For this review, take the finished solid that the model builds, in its own axes (mm). A direction names the side the tool comes from. Round coordinates to 2 decimals unless told otherwise and drop trailing zeros. Order: outer loops, then holes, each group sorted by start corner. A loop starts at its lowest first (then second) coordinate and runs counter-clockwise, first axis right, second up. Notation, with made-up numbers: (36, 85) -> (70, 85) arc R34 ccw to (70, 115) -> close; hole circle Ø4 at (-27.75, 73.5). An arc over 180 degrees is marked (long way). Use a Markdown table: item, result. Add a question column.
1) Consider section A-A (y = 7.5). State the section outline as (x, z) points (3 decimals).
2) Machinability: for faces 1 (the face through (-12, 3, -4)), 2 (the face through (-7, 2, -6.542)), 3 (the face through (10.318, 2.217, -6.705)), 4 (the face through (12, 3, -4)), 5 (the face through (10.27, 0.72, -4.52)), which of the approach directions +Z, -Z, +X, -X, +Y, -Y give a long, thin tool a straight path to every point of the face, cutting with its end or side? Answer none if there is none.
3) Clearance check with flat-ended pins moving along their axes: P1, Ø1.1, axis at x = 7, z = -4.5, coming from the -Y side; P2, Ø0.7, axis at x = 8, y = 1, coming from the +Z side; P3, Ø4.5, axis at x = 10, z = -5.5, coming from the +Y side; P4, Ø1, axis at x = -6.5, z = -1, coming from the -Y side. State where each tip first meets the part, or that it passes through.
4) Wall thickness on line 1 along X through (y, z) = (2.25, 1.25) (3 decimals); line 2 along Y through (x, z) = (3.25, 3.25); line 3 along Z through (x, y) = (8.75, 1): over which ranges is each line inside the solid? List them lowest first. Write a range as [from, to].
5) Consider section B-B (z = -4.55). Give the number of separate pieces and of enclosed holes in the cut face, plus the area to 3 significant figures.
6) Draft analysis for pull direction Z (two halves, no side actions). For faces 6 (the face through (-7.93, 3.45, -1.26)), 7 (the face through (8, 1, -5.82)), 8 (the face through (-13.3, 1.5, -4.6)), state which applies: pulls with the +Z half, pulls with the -Z half, needs draft (parallel to the pull), parting line crosses it, or undercut.
7) Consider section C-C (z = 4). State the section outline as (x, y) points (3 decimals).
8) Consider section D-D (x = 2.25). State the section outline as (y, z) points, plus the area to 4 significant figures.
```python
from build123d import *

# Parameters (mm, degrees)
SKETCH1_W          = 15
SKETCH1_H          = 17.3
EXTRUDE1_DEPTH     = 11.5
SKETCH2_W          = 12.15
SKETCH2_H          = 10
EXTRUDE2_DEPTH     = 17.3
EXTRUDE3_DEPTH     = 3
CUT_EXTRUDE3_DEPTH = 1.5875
CUT_EXTRUDE1_DEPTH = 18.998958303
FILLET3_R          = 1.5
FILLET1_R          = 1.5


with BuildPart() as part:
    # Sketch1 → Extrude1 (new body)
    with BuildSketch(Plane(origin=(0, 0, 0), x_dir=(1, 0, 0), z_dir=(0, 1, 0))):
        Rectangle(SKETCH1_W, SKETCH1_H)
    extrude(amount=EXTRUDE1_DEPTH)

    # Sketch2 → Extrude2 (cut)
    with BuildSketch(Plane.XY.offset(8.65)):
        with Locations((0, 5)):
            Rectangle(SKETCH2_W, SKETCH2_H)
    extrude(amount=-EXTRUDE2_DEPTH, mode=Mode.SUBTRACT)

    # Sketch3 → Extrude3 (add)
    with BuildSketch(Plane.XZ):
        with BuildLine():
            Line((7.5, -8.65), (10.169151464, -8.65))
            ThreePointArc((10.169151464, -8.65), (13.3, -4.55), (10.169151464, -0.45))
            Line((10.169151464, -0.45), (7.5, -0.45))
            Line((7.5, -0.45), (7.5, -8.65))
        make_face()
    extrude3 = extrude(amount=-EXTRUDE3_DEPTH)

    # Sketch8 → Cut-Extrude3 (cut)
    with BuildSketch(Plane(origin=(0, 3, 0), x_dir=(-1, 0, 0), z_dir=(0, 1, 0))):
        Polygon((-11.55, -5.993375673), (-9.05, -7.436751346), (-6.55, -5.993375673), (-6.55, -3.106624327), (-9.05, -1.663248654), (-11.55, -3.106624327), align=None)
    cut_extrude3 = extrude(amount=-CUT_EXTRUDE3_DEPTH, mode=Mode.SUBTRACT)

    # Sketch5 → Cut-Extrude1 (cut, through all)
    with BuildSketch(Plane.XZ.offset(-3)):
        with BuildLine():
            Line((9, -5.82), (7.5, -5.82))
            Line((7.5, -5.82), (7.5, -6.541858429))
            Line((7.5, -6.541858429), (6.075, -6.541858429))
            Line((6.075, -6.541858429), (6.075, -2.558141571))
            Line((6.075, -2.558141571), (7.5, -2.558141571))
            Line((7.5, -2.558141571), (7.5, -3.28))
            Line((7.5, -3.28), (9, -3.28))
            ThreePointArc((9, -3.28), (10.27, -4.55), (9, -5.82))
        make_face()
    cut_extrude1 = extrude(amount=CUT_EXTRUDE1_DEPTH, mode=Mode.SUBTRACT)

    # Mirror3: Extrude3, Cut-Extrude3, Cut-Extrude1 across plane
    add(extrude3.mirror(Plane(origin=(0, 0, 0), x_dir=(0, 0, 1), z_dir=(1, 0, 0))))
    add(cut_extrude3.mirror(Plane(origin=(0, 0, 0), x_dir=(0, 0, 1), z_dir=(1, 0, 0))), mode=Mode.SUBTRACT)
    add(cut_extrude1.mirror(Plane(origin=(0, 0, 0), x_dir=(0, 0, 1), z_dir=(1, 0, 0))), mode=Mode.SUBTRACT)

    # Fillet3
    fillet3_edges = [part.edges().sort_by_distance(p)[0] for p in [
        (-7.5, 11.5, 0),
        (7.5, 11.5, 0),
    ]]
    fillet(fillet3_edges, radius=FILLET3_R)

    # Fillet1
    # the kernel refuses this fillet: 1.5 mm, written as the material it adds along each edge
    with BuildSketch(Plane(origin=(7.5, 3, -0.45), x_dir=(0, 1, 0), z_dir=(0, 0, -1))) as fillet1_piece_1_section:
        with BuildLine():
            CenterArc((FILLET1_R, FILLET1_R), FILLET1_R, 180, 90)
            Line((0, FILLET1_R), (0, 0))
            Line((0, 0), (FILLET1_R, 0))
        make_face()
    fillet1_piece_1 = extrude(amount=5.858141571, mode=Mode.PRIVATE)
    fillet1_piece_1 = split(fillet1_piece_1, bisect_by=Plane(origin=(8.228724566, 3.349084614, -2.137412247), z_dir=(-0.5000000000000001, 0, 0.8660254037844386)), keep=Keep.TOP, mode=Mode.PRIVATE)
    add(fillet1_piece_1)
    with BuildSketch(Plane(origin=(7.5, 3, -2.791858429), x_dir=(0, 1, 0), z_dir=(0, 0, -1))) as fillet1_piece_2_section:
        with BuildLine():
            CenterArc((FILLET1_R, FILLET1_R), FILLET1_R, 180, 90)
            Line((0, FILLET1_R), (0, 0))
            Line((0, 0), (FILLET1_R, 0))
        make_face()
    fillet1_piece_2 = extrude(amount=5.858141571, mode=Mode.PRIVATE)
    fillet1_piece_2 = split(fillet1_piece_2, bisect_by=Plane(origin=(8.228724566, 3.349084614, -6.962587753), z_dir=(-0.5000000000000002, 0, -0.8660254037844386)), keep=Keep.TOP, mode=Mode.PRIVATE)
    add(fillet1_piece_2)
    with BuildSketch(Plane(origin=(-7.5, 3, -2.791858429), x_dir=(0, 1, 0), z_dir=(0, 0, -1))) as fillet1_piece_3_section:
        with BuildLine():
            CenterArc((FILLET1_R, -FILLET1_R), FILLET1_R, 90, 90)
            Line((0, -FILLET1_R), (0, 0))
            Line((0, 0), (FILLET1_R, 0))
        make_face()
    fillet1_piece_3 = extrude(amount=5.858141571, mode=Mode.PRIVATE)
    fillet1_piece_3 = split(fillet1_piece_3, bisect_by=Plane(origin=(-8.228724566, 3.349084614, -6.962587753), z_dir=(0.5000000000000002, 0, -0.8660254037844386)), keep=Keep.TOP, mode=Mode.PRIVATE)
    add(fillet1_piece_3)
    with BuildSketch(Plane(origin=(-7.5, 3, -0.45), x_dir=(0, 1, 0), z_dir=(0, 0, -1))) as fillet1_piece_4_section:
        with BuildLine():
            CenterArc((FILLET1_R, -FILLET1_R), FILLET1_R, 90, 90)
            Line((0, -FILLET1_R), (0, 0))
            Line((0, 0), (FILLET1_R, 0))
        make_face()
    fillet1_piece_4 = extrude(amount=5.858141571, mode=Mode.PRIVATE)
    fillet1_piece_4 = split(fillet1_piece_4, bisect_by=Plane(origin=(-8.228724566, 3.349084614, -2.137412247), z_dir=(0.5000000000000001, 0, 0.8660254037844386)), keep=Keep.TOP, mode=Mode.PRIVATE)
    add(fillet1_piece_4)


solid = part.part
```
Results list:
| question | item | result |
|---|---|---|
| 1 | outline | (-7.5, -8.65) -> (-6.075, -8.65) -> (-6.075, 8.65) -> (-7.5, 8.65) -> close; (6.075, -8.65) -> (7.5, -8.65) -> (7.5, 8.65) -> (6.075, 8.65) -> close |
| 2 | face 1 | +Z, -Z, -X, +Y |
| 2 | face 2 | -Y |
| 2 | face 3 | +Y |
| 2 | face 4 | +Z, -Z, +X, +Y |
| 2 | face 5 | +Y, -Y |
| 3 | P1 | y = 3 |
| 3 | P2 | z = -0.45 |
| 3 | P3 | y = 3.15 |
| 3 | P4 | y = 0 |
| 4 | line 1 | [-7.5, -6.075], [6.075, 7.5] |
| 4 | line 2 | [10, 11.5] |
| 4 | line 3 | [-8.65, -5.82], [-3.28, -0.45] |
| 5 | separate pieces | 3 |
| 5 | enclosed holes | 0 |
| 5 | area | 55.6 mm2 |
| 6 | face 6 | needs draft |
| 6 | face 7 | undercut |
| 6 | face 8 | parting line crosses it |
| 7 | outline | (-7.5, 0) -> (-6.075, 0) -> (-6.075, 10) -> (6.075, 10) -> (6.075, 0) -> (7.5, 0) -> (7.5, 10) arc R1.5 ccw to (6, 11.5) -> (-6, 11.5) arc R1.5 ccw to (-7.5, 10) -> close |
| 8 | outline | (10, -8.65) -> (11.5, -8.65) -> (11.5, 8.65) -> (10, 8.65) -> close |
| 8 | area | 25.95 mm2 |
